from build123d import *

# Parameters (mm, degrees)
SKETCH1_W           = 10
SKETCH1_H           = 5
SKETCH1_W_2         = 9.935990319
SKETCH1_W_3         = 10.064009681
BOSS_EXTRUDE1_DEPTH = 5


with BuildPart() as part:
    # Sketch1 → Boss-Extrude1 (new body)
    with BuildSketch(Plane.XY):
        with BuildLine():
            Line((44.999999787, 7.5), (44.999999787, 30.5))
            ThreePointArc((44.999999787, 30.5), (44.41421335, 31.914213562), (42.999999787, 32.5))
            Line((42.999999787, 32.5), (14.260362516, 32.5))
            ThreePointArc((14.260362516, 32.5), (12.846148953, 31.914213562), (12.260362516, 30.5))
            Line((12.260362516, 30.5), (12.260362516, 7.356217509))
            ThreePointArc((12.260362516, 7.356217509), (12.125280096, 6.734124269), (11.744362516, 6.224076175))
            ThreePointArc((11.744362516, 6.224076175), (11.490417462, 5.884044113), (11.400362516, 5.469315286))
            Line((11.400362516, 5.469315286), (11.400362516, -5.143782491))
            Line((11.400362516, -5.143782491), (-10.599637484, -5.143782491))
            Line((-10.599637484, -5.143782491), (-10.599637484, 4.856217509))
            ThreePointArc((-10.599637484, 4.856217509), (-10.892530703, 5.563324291), (-11.599637484, 5.856217509))
            Line((-11.599637484, 5.856217509), (-14.070705683, 5.856217509))
            ThreePointArc((-14.070705683, 5.856217509), (-15.484919246, 5.270431072), (-16.070705683, 3.856217509))
            Line((-16.070705683, 3.856217509), (-16.070705683, -13.143782491))
            ThreePointArc((-16.070705683, -13.143782491), (-15.484919246, -14.557996053), (-14.070705683, -15.143782491))
            Line((-14.070705683, -15.143782491), (21.781895091, -15.143782491))
            ThreePointArc((21.781895091, -15.143782491), (25.832683233, -14.286600187), (29.189018592, -11.862005577))
            Line((29.189018592, -11.862005577), (43.703561538, 4.140888457))
            ThreePointArc((43.703561538, 4.140888457), (44.664643865, 5.699695686), (44.999999787, 7.5))
        make_face()
        with Locations((20.760362516, 25)):
            Rectangle(SKETCH1_W, SKETCH1_H, mode=Mode.SUBTRACT)
        with Locations((20.792367357, 14.995460919)):
            Rectangle(SKETCH1_W_2, SKETCH1_H, mode=Mode.SUBTRACT)
        with Locations((35.760362516, 25)):
            Rectangle(SKETCH1_W, SKETCH1_H, mode=Mode.SUBTRACT)
        with Locations((35.792367357, 14.995460919)):
            Rectangle(SKETCH1_W_3, SKETCH1_H, mode=Mode.SUBTRACT)
    extrude(amount=BOSS_EXTRUDE1_DEPTH)


solid = part.part
Model file for the job. Use its own axes, mm. A direction names the side the tool comes from. Give positions to 0.01 mm unless a question says otherwise; leave off trailing zeros. Order: outer loops, then holes, each group sorted by start corner. A loop starts at its lowest first (then second) coordinate and runs counter-clockwise, first axis right, second up. Notation, with made-up numbers: M 80,41 L 137,41 A24 ccw 137,62 Z; hole C 89.25,-4 d6. An arc over 180 degrees is marked long. Put each result on its own line as item: value. Start each with the question number.
(1) Band-saw the part on B-B on y = -4.5. Give the cut face in (x, z).
(2) Band-saw the part on C-C on z = 4. Count the separate pieces of the cut face and the enclosed holes in it, then the cut area to 3 significant figures.
(3) Pull direction X, two halves, no side cores. Call faces 1 (the face through (29, 32.5, 2)), 2 (the face through (40.76, 25, 2)), 3 (the face through (44.655, 5.676, 2.465)): released by +X, released by -X, zero draft, split by the parting line, or undercut.
(4) Band-saw the part on D-D on x = 33.5. Give the cut face in (y, z), then the cut area to 3 significant figures.
(5) Pin check, flat tips, straight feed: pin 1 Ø1.5 at (y, z) = (24.5, 2.5) entering from -X; pin 2 Ø2 at (x, z) = (-12.5, 3.5) entering from +Y; pin 3 Ø2.5 at (y, z) = (1, 2.5) entering from +X. Stop position of each tip, or through.
(6) Band-saw the part on A-A on x = 21. Give the cut face in (y, z), then the cut area to 3 significant figures.
(7) Tool access for faces 4 (the face through (-13, 5.856, 2)), 5 (the face through (30.76, 15, 2)), 6 (the face through (21, 9, 0)), 7 (the face through (-10.6, 0, 2)), 8 (the face through (-16.071, -5, 2)): list every direction of +Z, -Z, +X, -X, +Y, -Y with a clear straight run to the whole face (end or side of a thin tool).
(8) Drill centre lines: L1, parallel to X at y = 24, z = 1.7; L2, parallel to Y at x = 19, z = 3.85; L3, parallel to Y at x = 34, z = 0.9. Where is each one in solid material? Low to high. Write a range as [from, to].
Results below:
1. outline: M -16.07,0 L -10.6,0 L -10.6,5 L -16.07,5 Z; M 11.4,0 L 35.87,0 L 35.87,5 L 11.4,5 Z
2. separate pieces: 1
2. enclosed holes: 4
2. area: 1,510 mm2
3. face 1: zero draft
3. face 2: undercut
3. face 3: released by +X
4. outline: M -7.11,0 L 12.5,0 L 12.5,5 L -7.11,5 Z; M 17.5,0 L 22.5,0 L 22.5,5 L 17.5,5 Z; M 27.5,0 L 32.5,0 L 32.5,5 L 27.5,5 Z
4. area: 148 mm2
5. pin 1: stops at x = 12.26
5. pin 2: stops at y = 5.86
5. pin 3: stops at x = 41.99
6. outline: M -15.14,0 L 12.5,0 L 12.5,5 L -15.14,5 Z; M 17.5,0 L 22.5,0 L 22.5,5 L 17.5,5 Z; M 27.5,0 L 32.5,0 L 32.5,5 L 27.5,5 Z
6. area: 188 mm2
7. face 4: +Z, -Z, -X, +Y
7. face 5: +Z, -Z
7. face 6: -Z, +X, -X, +Y, -Y
7. face 7: +Z, -Z, +Y
7. face 8: +Z, -Z, -X, +Y, -Y
8. L1: x = [12.26, 15.76], [25.76, 30.76], [40.76, 45]
8. L2: y = [-15.14, 12.5], [17.5, 22.5], [27.5, 32.5]
8. L3: y = [-6.56, 12.5], [17.5, 22.5], [27.5, 32.5]
